Here's how the part is built. I have some questions about the finished solid (model axes, mm). A direction names the side the tool comes from. Coordinates: 2 decimals unless noted, no trailing zeros. Write each loop counter-clockwise with the first axis right and the second up, starting at its lowest first coordinate (ties: lowest second). Pieces come first, ordered by that corner, then holes. Notation, with made-up numbers: (-10.5, 63.5) -> (30.5, 63.5) arc R21 cw to (30.5, 74.5) -> close; hole circle Ø7 at (-9.75, 85.5). An arc over 180 degrees is marked (long way). Use a Markdown table: item, result. Add a question column.
Item 1: On a 3-axis mill with a long thin cutter (end or side, diameter ignored), from which of +Z, -Z, +X, -X, +Y, -Y can I reach the whole of each face in a straight line? I mean faces 4 (the flat face through (-5, 0, 22.7)), 5 (the flat face through (2, 0, 26.7)), 6 (the flat face through (10, -5, 22.7)), 7 (the flat face through (-12.5, 0.1, 15.9)). Say none if no direction works.
Item 2: Will these pins go through, and if not, where does the flat tip stop? pin 1 Ø0.8 at (x, z) = (-0.5, 24.5) entering from -Y; pin 2 Ø3 at (x, y) = (7.5, 4) entering from +Z; pin 3 Ø5 at (x, y) = (-14.5, 3) entering from -Z.
Item 3: Imagine slicing it at B-B, the plane z = 26.25. Write out the boundary of the cut face in (x, y) (3 decimals), and give its area (3 significant figures).
Item 4: Imagine slicing it at D-D, the plane x = -8. Write out the boundary of the cut face in (y, z).
Item 5: If we mould it in two halves opening along Y, with no side actions, what happens to faces 1 (the flat face through (15, 0.638, 17)), 2 (the flat face through (0, 5.9, 11)), 3 (the flat face through (5, 0, 29.9))? For each: pulls with the +Y half, pulls with the -Y half, needs draft (parallel to the pull), parting line crosses it, or undercut.
Item 6: If I drill on line 1 along Y through (x, z) = (13.65, 17.1); line 2 along Z through (x, y) = (-1.5, -0.75); line 3 along X through (y, z) = (4.75, 2.5), over which ranges is the centre line in solid material (lowest first)? Write a range as from..to.
Item 7: Imagine slicing it at C-C, the plane y = -5. Write out the boundary of the cut face in (x, z).
Item 8: Imagine slicing it at A-A, the plane x = 13.65. Write out the boundary of the cut face in (y, z), and give its area (3 significant figures).
```python
from build123d import *

# Parameters (mm, degrees)
F0_W      = 22.5
F0_H      = 11.8
F1_DEPTH  = 22.7
F2_W      = 11.8
F2_H      = 2.5
F3_DEPTH  = 4.7
F4_W      = 11.8
F4_H      = 2.5
F5_DEPTH  = 4.7
F7_DEPTH  = 2.5
F9_DEPTH  = 2.5
F10_R     = 2.3
F11_DEPTH = 4
F12_DEPTH = 7.2


with BuildPart() as f1:
    # F0 (on Top) → F1 (new body)
    with BuildSketch(Plane.XY):
        Rectangle(F0_W, F0_H)
    extrude(amount=F1_DEPTH)

    # F2 (on face) → F3 (join)
    with BuildSketch(Plane(origin=(-11.25, 0, 0), x_dir=(0, -1, 0), z_dir=(-1, 0, 0))):
        with Locations((0, 17.15)):
            Rectangle(F2_W, F2_H)
    extrude(amount=F3_DEPTH)

    # F4 (on face) → F5 (join)
    with BuildSketch(Plane.YZ.offset(11.25)):
        with Locations((0, 17.15)):
            Rectangle(F4_W, F4_H)
    extrude(amount=F5_DEPTH)

    # F6 (on face) → F7 (cut)
    with BuildSketch(Plane.XY.offset(18.4)):
        with BuildLine():
            Line((-15.95, 0.65), (-15.95, 0))
            Line((-15.95, 0), (-14.65, 0))
            ThreePointArc((-14.65, 0), (-14.5880656181, 0.3464576398), (-14.4099342077, 0.65))
            Line((-14.4099342077, 0.65), (-15.95, 0.65))
        make_face()
        with BuildLine():
            Line((-14.65, 0), (-15.95, 0))
            Line((-15.95, 0), (-15.95, -0.65))
            Line((-15.95, -0.65), (-14.4099342077, -0.65))
            ThreePointArc((-14.4099342077, -0.65), (-14.5880656181, -0.3464576398), (-14.65, 0))
        make_face()
        with BuildLine():
            ThreePointArc((-14.4099342077, 0.65), (-14.5880656181, 0.3464576398), (-14.65, 0))
            ThreePointArc((-14.65, 0), (-14.5880656181, -0.3464576398), (-14.4099342077, -0.65))
            ThreePointArc((-14.4099342077, -0.65), (-13.3035423602, -0.9380656181), (-12.65, 0))
            ThreePointArc((-12.65, 0), (-13.3035423602, 0.9380656181), (-14.4099342077, 0.65))
        make_face()
    extrude(amount=-F7_DEPTH, mode=Mode.SUBTRACT)

    # F8 (on face) → F9 (cut)
    with BuildSketch(Plane.XY.offset(18.4)):
        with BuildLine():
            Line((15.95, -0.6616220634), (15.95, 0))
            Line((15.95, 0), (14.65, 0))
            ThreePointArc((14.65, 0), (14.5853709102, -0.3536682915), (14.3998374792, -0.6616220634))
            Line((14.3998374792, -0.6616220634), (15.95, -0.6616220634))
        make_face()
        with BuildLine():
            Line((14.65, 0), (15.95, 0))
            Line((15.95, 0), (15.95, 0.6383779366))
            Line((15.95, 0.6383779366), (14.4197230736, 0.6383779366))
            ThreePointArc((14.4197230736, 0.6383779366), (14.5906707909, 0.3393205906), (14.65, 0))
        make_face()
        with BuildLine():
            ThreePointArc((14.3998374792, -0.6616220634), (14.5853709102, -0.3536682915), (14.65, 0))
            ThreePointArc((14.65, 0), (14.5906707909, 0.3393205906), (14.4197230736, 0.6383779366))
            ThreePointArc((14.4197230736, 0.6383779366), (12.6501169726, 0.0152948218), (14.3998374792, -0.6616220634))
        make_face()
    extrude(amount=-F9_DEPTH, mode=Mode.SUBTRACT)

    # F10 (on face) → F11 (join)
    with BuildSketch(Plane.XY.offset(22.7)):
        with BuildLine():
            ThreePointArc((0.0058443136, -2.5), (6.6305236137, -5.759362749), (11.25, 0))
            ThreePointArc((11.25, 0), (6.6259878855, 5.7603693385), (0.0019135878, 2.4915801668))
            ThreePointArc((0.0019135878, 2.4915801668), (-0.0329189996, 2.415405358), (-0.0666666667, 2.3387437274))
            ThreePointArc((-0.0666666667, 2.3387437274), (1.1064937799, 1.4215601758), (1.55, 0))
            ThreePointArc((1.55, 0), (1.1064937799, -1.4215601758), (-0.0666666667, -2.3387437274))
            ThreePointArc((-0.0666666667, -2.3387437274), (-0.031015269, -2.4196435017), (0.0058443136, -2.5))
        make_face()
        with Locations((5.35, 0)):
            Circle(F10_R, mode=Mode.SUBTRACT)
        with BuildLine():
            ThreePointArc((-0.0666666667, 2.3387437274), (-0.0329189996, 2.415405358), (0.0019135878, 2.4915801668))
            Line((0.0019135878, 2.4915801668), (-0.7449920185, 2.4915801668))
            ThreePointArc((-0.7449920185, 2.4915801668), (-0.4004898102, 2.4388600926), (-0.0666666667, 2.3387437274))
        make_face()
        with BuildLine():
            Line((-0.95, -2.5), (0.0058443136, -2.5))
            ThreePointArc((0.0058443136, -2.5), (-0.031015269, -2.4196435017), (-0.0666666667, -2.3387437274))
            ThreePointArc((-0.0666666667, -2.3387437274), (-0.5010341429, -2.4593555374), (-0.95, -2.5))
        make_face()
        with BuildLine():
            ThreePointArc((-0.0666666667, -2.3387437274), (-0.55, 0), (-0.0666666667, 2.3387437274))
            ThreePointArc((-0.0666666667, 2.3387437274), (-0.4004898102, 2.4388600926), (-0.7449920185, 2.4915801668))
            Line((-0.7449920185, 2.4915801668), (-1.1550079815, 2.4915801668))
            ThreePointArc((-1.1550079815, 2.4915801668), (-3.4478941548, -0.1025904066), (-0.95, -2.5))
            ThreePointArc((-0.95, -2.5), (-0.5010341429, -2.4593555374), (-0.0666666667, -2.3387437274))
        make_face()
        with BuildLine():
            Line((-1.1550079815, 2.4915801668), (-0.7449920185, 2.4915801668))
            ThreePointArc((-0.7449920185, 2.4915801668), (-0.95, 2.5), (-1.1550079815, 2.4915801668))
        make_face()
        with BuildLine():
            ThreePointArc((5.3500000048, -5.9), (9.5219300107, -4.1719300073), (11.25, 0))
            ThreePointArc((11.25, 0), (9.521930009, 4.171930009), (5.35, 5.9))
            ThreePointArc((5.35, 5.9), (2.1790634652, 4.975455908), (0.0019135878, 2.4915801668))
            ThreePointArc((0.0019135878, 2.4915801668), (-0.0329189996, 2.415405358), (-0.0666666667, 2.3387437274))
            ThreePointArc((-0.0666666667, 2.3387437274), (1.1064937799, 1.4215601758), (1.55, 0))
            ThreePointArc((1.55, 0), (1.1064937799, -1.4215601758), (-0.0666666667, -2.3387437274))
            ThreePointArc((-0.0666666667, -2.3387437274), (-0.031015269, -2.4196435017), (0.0058443136, -2.5))
            ThreePointArc((0.0058443136, -2.5), (2.1829824776, -4.9779513872), (5.3500000048, -5.9))
        make_face()
        with Locations((5.35, 0)):
            Circle(F10_R, mode=Mode.SUBTRACT)
        with BuildLine():
            ThreePointArc((1.55, 0), (1.1064937799, 1.4215601758), (-0.0666666667, 2.3387437274))
            ThreePointArc((-0.0666666667, 2.3387437274), (-0.55, 0), (-0.0666666667, -2.3387437274))
            ThreePointArc((-0.0666666667, -2.3387437274), (1.1064937799, -1.4215601758), (1.55, 0))
        make_face()
    extrude(amount=F11_DEPTH)

    # F12 (add): a face of the model
    f12_faces = [f1.faces().sort_by_distance(p)[0] for p in [
        (5.35, 0, 22.7),
    ]]
    extrude(f12_faces, amount=F12_DEPTH)


solid = f1.part
```
Ans:
| question | item | result |
|---|---|---|
| 1 | face 4 | +Z, -X |
| 1 | face 5 | +Z |
| 1 | face 6 | +Z, +X, -Y |
| 1 | face 7 | -Z, -X, +Y, -Y |
| 2 | pin 1 | stops at y = -2.5 |
| 2 | pin 2 | stops at z = 26.7 |
| 2 | pin 3 | stops at z = 15.9 |
| 3 | outline | (-0.95, -2.5) -> (0.006, -2.5) arc R5.9 ccw (long way) to (0.002, 2.492) -> (-0.745, 2.492) arc R2.5 ccw (long way) to start |
| 3 | area | 122 mm^2 |
| 4 | outline | (-5.9, 0) -> (5.9, 0) -> (5.9, 22.7) -> (-5.9, 22.7) -> close |
| 5 | face 1 | undercut |
| 5 | face 2 | pulls with the +Y half |
| 5 | face 3 | needs draft |
| 6 | line 1 | y = -5.9..-1, 1..5.9 |
| 6 | line 2 | z = 0..26.7 |
| 6 | line 3 | x = -11.25..11.25 |
| 7 | outline | (-15.95, 15.9) -> (-11.25, 15.9) -> (-11.25, 0) -> (11.25, 0) -> (11.25, 15.9) -> (15.95, 15.9) -> (15.95, 18.4) -> (11.25, 18.4) -> (11.25, 22.7) -> (8.48, 22.7) -> (8.48, 26.7) -> (2.22, 26.7) -> (2.22, 22.7) -> (-11.25, 22.7) -> (-11.25, 18.4) -> (-15.95, 18.4) -> close |
| 8 | outline | (-5.9, 15.9) -> (-1, 15.9) -> (-1, 18.4) -> (-5.9, 18.4) -> close; (1, 15.9) -> (5.9, 15.9) -> (5.9, 18.4) -> (1, 18.4) -> close |
| 8 | area | 24.5 mm^2 |
